```python
from build123d import *

# Parameters (mm, degrees)
F2_R     = 7.5
F3_DEPTH = 33


with BuildPart() as f1:
    # F0 (on Right) → F1 (revolve)
    with BuildSketch(Plane.YZ):
        with BuildLine():
            Line((3, 32), (3, 0))
            Line((3, 0), (24, 0))
            Line((24, 0), (24, 26))
            Line((24, 26), (66, 26))
            Line((66, 26), (66, 29))
            Line((66, 29), (93, 30.3359316767))
            Line((93, 30.3359316767), (93, 38.3359316767))
            Line((93, 38.3359316767), (85, 38.3359316767))
            Line((85, 38.3359316767), (85, 45))
            Line((85, 45), (55, 45))
            Line((55, 45), (55, 38.3359316767))
            Line((55, 38.3359316767), (55, 33.1562738389))
            ThreePointArc((55, 33.1562738389), (52.5710475058, 28.8679507724), (47.6441141108, 28.7460809092))
            Line((47.6441141108, 28.7460809092), (33, 39))
            Line((33, 39), (0, 39))
            Line((0, 39), (0, 32))
            Line((0, 32), (3, 32))
        make_face()
    revolve(axis=Axis((0, 13.5, 0), (0, 1, 0)))

    # F2 (on face) → F3 (join)
    with BuildSketch(Plane.XZ):
        with BuildLine():
            Line((36.6079755837, 13.4482758621), (17.8346547716, 64.5517241379))
            ThreePointArc((17.8346547716, 64.5517241379), (0, 77), (-17.8346547716, 64.5517241379))
            Line((-17.8346547716, 64.5517241379), (-36.6079755837, 13.4482758621))
            ThreePointArc((-36.6079755837, 13.4482758621), (-22.3217073874, 31.980328005), (0, 39))
            ThreePointArc((0, 39), (22.3217073874, 31.980328005), (36.6079755837, 13.4482758621))
        make_face()
        with Locations((0, 58)):
            Circle(F2_R, mode=Mode.SUBTRACT)
        with BuildLine():
            ThreePointArc((36.6079755837, -13.4482758621), (0, -39), (-36.6079755837, -13.4482758621))
            Line((-36.6079755837, -13.4482758621), (-17.8346547716, -64.5517241379))
            ThreePointArc((-17.8346547716, -64.5517241379), (0, -77), (17.8346547716, -64.5517241379))
            Line((17.8346547716, -64.5517241379), (36.6079755837, -13.4482758621))
        make_face()
        with Locations((0, -58)):
            Circle(F2_R, mode=Mode.SUBTRACT)
    extrude(amount=-F3_DEPTH)


solid = f1.part
```
For this review, take the finished solid that the model builds, in its own axes (mm). A direction names the side the tool comes from. Round coordinates to 2 decimals unless told otherwise and drop trailing zeros. Order: outer loops, then holes, each group sorted by start corner. A loop starts at its lowest first (then second) coordinate and runs counter-clockwise, first axis right, second up.
Q1. Mouldability with a two-part tool opening along Z and no side actions: class faces 1 (the cylindrical face through (0, 16, 77)), 2 (the conical face through (-18.06, 79.69, -23.55)), 3 (the cylindrical face through (39, 16, 0)) as pulls with the +Z half, pulls with the -Z half, needs draft (parallel to the pull), parting line crosses it, or undercut.
Findings below:
face 1: pulls with the +Z half
face 2: undercut
face 3: parting line crosses it
Q2. We need section B-B, the plane z = -58. Give the boundary of the cut face in (x, y).
Findings below:
outline: (-20.24, 0) - (-7.5, 0) - (-7.5, 33) - (-20.24, 33) - close; (7.5, 0) - (20.24, 0) - (20.24, 33) - (7.5, 33) - close
Q3. Insertion check: P1, Ø10, axis at x = 13, z = 6, coming from the -Y side; P2, Ø15.5, axis at x = -1.5, z = -10.5, coming from the +Y side; P3, Ø10, axis at y = 22.5, z = 23, coming from the +X side; P4, Ø13.5, axis at x = 0, z = -58, coming from the -Y side. Each pin has a flat end and moves straight along its axis. Give the tip position at first contact, or say it passes through.
Findings below:
P1: stops at y = 3
P2: stops at y = 24
P3: stops at x = 34.94
P4: passes through
Q4. Wall thickness on line 1 (Y direction, x = 6, z = -40.5); line 2 (Y direction, x = -19, z = -41); line 3 (X direction, y = 54, z = 0): over which ranges is each line inside the solid? List them lowest first.
Findings below:
line 1: y = 0 to 33, 55 to 85
line 2: y = 0 to 33
line 3: x = -30.16 to -26, 26 to 30.16
Q5. We need section D-D, the plane x = 0. State how many separate pieces and enclosed holes the cut face has, plus the area to 3 significant figures.
Findings below:
separate pieces: 3
enclosed holes: 0
area: 4,850 mm2
Q6. Machinability: for faces 4 (the flat face through (27.353, 16.269, 38.642)), 5 (the flat face through (27.09, 16.27, -39.36)), 6 (the flat face through (0, 3, 0)), which of the approach directions +Z, -Z, +X, -X, +Y, -Y give a long, thin tool a straight path to every point of the face, cutting with its end or side? Answer none if there is none.
Findings below:
face 4: +Z, +X, -Y
face 5: -Z, +X, -Y
face 6: -Y
Q7. We need section A-A, the plane y = 20. Give the boundary of the cut face in (x, z), plus the area to 3 significant figures.
Findings below:
outline: (-36.61, -13.45) - (-17.83, -64.55) arc R19 ccw to (17.83, -64.55) - (36.61, -13.45) arc R39 ccw to (36.61, 13.45) - (17.83, 64.55) arc R19 ccw to (-17.83, 64.55) - (-36.61, 13.45) arc R39 ccw to start; hole circle Ø15 at (0, -58); hole circle Ø15 at (0, 58)
area: 7,910 mm2
Q8. We need section C-C, the plane z = 0. Give the boundary of the cut face in (x, y).
Findings below:
outline: (-45, 55) - (-33.16, 55) arc R5 cw to (-28.75, 47.64) - (-39, 33) - (-39, 0) - (-32, 0) - (-32, 3) - (32, 3) - (32, 0) - (39, 0) - (39, 33) - (28.75, 47.64) arc R5 cw to (33.16, 55) - (45, 55) - (45, 85) - (38.34, 85) - (38.34, 93) - (30.34, 93) - (29, 66) - (26, 66) - (26, 24) - (-26, 24) - (-26, 66) - (-29, 66) - (-30.34, 93) - (-38.34, 93) - (-38.34, 85) - (-45, 85) - close
